from build123d import *

# Parameters (mm, degrees)
SKETCH_1_R               = 2
EXTRUDE_1_DEPTH          = 16
EXTRUDE_2_DEPTH          = 3
SKETCH_4_R               = 3.15
CUT_EXTRUDE_6_DEPTH      = 2.5
FILLET_3_R               = 0.6
SKETCH_7_R               = 3.175
EXTRUDE_3_DEPTH          = 1.4
CUT_EXTRUDE_9_DEPTH      = 1
CUT_EXTRUDE_9_DEPTH_BACK = 26
FILLET_6_R               = 1
EXTRUDE_5_DEPTH          = 3
FILLET_7_R               = 0.3
CUT_EXTRUDE_10_REACH     = 2.675
SKETCH_13_R              = 1.8
CUT_EXTRUDE_11_REACH     = 18
SKETCH_14_W              = 2.079062288
SKETCH_14_H              = 0.49177122


with BuildPart() as part:
    # Sketch 1 → Extrude 1 (new body)
    with BuildSketch(Plane(origin=(0, 0, 0), x_dir=(1, 0, 0), z_dir=(0, 1, 0))):
        Circle(SKETCH_1_R)
    extrude(amount=EXTRUDE_1_DEPTH)

    # Fillet 3
    fillet_3_edges = [part.edges().sort_by_distance(p)[0] for p in [
        (-2, 0, 0),
    ]]
    fillet(fillet_3_edges, radius=FILLET_3_R)

    # Sketch 7 → Extrude 3 (add)
    with BuildSketch(Plane(origin=(0, 16, 0), x_dir=(1, 0, 0), z_dir=(0, 1, 0))):
        Circle(SKETCH_7_R)
    extrude(amount=-EXTRUDE_3_DEPTH)

    # Sketch 10 → Cut-Extrude 9 (cut, two sides)
    with BuildSketch(Plane.XZ) as cut_extrude_9_sk:
        with BuildLine():
            Line((-1.307669683, 0.5), (1.307669683, 0.5))
            ThreePointArc((1.307669683, 0.5), (0, -1.4), (-1.307669683, 0.5))
        make_face()
    extrude(amount=CUT_EXTRUDE_9_DEPTH, mode=Mode.SUBTRACT)
    extrude(cut_extrude_9_sk.sketch, amount=-CUT_EXTRUDE_9_DEPTH_BACK, mode=Mode.SUBTRACT)

    # Fillet 6
    fillet_6_edges = [part.edges().sort_by_distance(p)[0] for p in [
        (0, 16, -1.4),
    ]]
    fillet(fillet_6_edges, radius=FILLET_6_R)



with BuildPart() as body_2:
    # Sketch 2 → Extrude 2 (new body)
    with BuildSketch(Plane.XY):
        with BuildLine():
            ThreePointArc((4.245738578, 21.991208882), (-3.671541908, 23.101880092), (0, 16))
            ThreePointArc((0, 16), (3.671541908, 17.898119908), (4.245738578, 21.991208882))
        make_face()
    extrude(amount=EXTRUDE_2_DEPTH)

    # Sketch 4 → Cut-Extrude 6 (cut)
    with BuildSketch(Plane(origin=(0, 0, 0), x_dir=(-1, 0, 0), z_dir=(0, 0, -1))):
        with Locations((0, 20.5)):
            Circle(SKETCH_4_R)
    extrude(amount=-CUT_EXTRUDE_6_DEPTH, mode=Mode.SUBTRACT)


with BuildPart() as part_1:
    add(part.part)

    add(body_2.part)  # Extrude 5 merges body 2
    # Sketch 12 → Extrude 5 (add)
    with BuildSketch(Plane.XY.offset(3)):
        with BuildLine():
            Line((-3.175, 16), (-4.239526881, 18.991221744))
            ThreePointArc((-4.239526881, 18.991221744), (0, 16), (4.239526881, 18.991221744))
            Line((4.239526881, 18.991221744), (3.175, 16))
            Line((3.175, 16), (3.175, 14.6))
            Line((3.175, 14.6), (-3.175, 14.6))
            Line((-3.175, 14.6), (-3.175, 16))
        make_face()
    extrude(amount=-EXTRUDE_5_DEPTH)

    # Fillet 7
    fillet_7_edges = [part_1.edges().sort_by_distance(p)[0] for p in [
        (3.15, 20.5, 0),
    ]]
    fillet(fillet_7_edges, radius=FILLET_7_R)

    # Sketch 13 → Cut-Extrude 10 (cut, up to next)
    with BuildSketch(Plane(origin=(0, 0, 2.5), x_dir=(-1, 0, 0), z_dir=(0, 0, -1)), mode=Mode.PRIVATE) as cut_extrude_10_sk1:
        with Locations((0, 20.5)):
            Circle(SKETCH_13_R)
    cut_extrude_10_tool1 = extrude(cut_extrude_10_sk1.sketch, amount=-CUT_EXTRUDE_10_REACH, mode=Mode.PRIVATE) & part_1.part
    add(cut_extrude_10_tool1.solids().sort_by_distance((0, 20.5, 2.5))[0], mode=Mode.SUBTRACT)

    # Sketch 14 → Cut-Extrude 11 (cut, up to next)
    with BuildSketch(Plane(origin=(0, 16, 0), x_dir=(1, 0, 0), z_dir=(0, 1, 0)), mode=Mode.PRIVATE) as cut_extrude_11_sk1:
        with Locations((0, -3.24588561)):
            Rectangle(SKETCH_14_W, SKETCH_14_H)
    cut_extrude_11_tool1 = extrude(cut_extrude_11_sk1.sketch, amount=-CUT_EXTRUDE_11_REACH, mode=Mode.PRIVATE) & part_1.part
    add(cut_extrude_11_tool1.solids().sort_by_distance((0, 16, 3.245886))[0], mode=Mode.SUBTRACT)


solid = part_1.part
Input: part model. Units: mm. Frame: model coordinates. A direction names the side the tool comes from. Give positions to 0.01 mm unless a question says otherwise; leave off trailing zeros. Order: outer loops, then holes, each group sorted by start corner. A loop starts at its lowest first (then second) coordinate and runs counter-clockwise, first axis right, second up. Notation, with made-up numbers: (-18, 12.5) -> (40, 12.5) arc R10 cw to (40, 21.5) -> close; hole circle Ø11 at (49.25, -0.75). An arc over 180 degrees is marked (long way). Use one line per item in the form item = value.
1) Section A-A, the plane x = 0. Return loops of the section in (y, z) (3 decimals).
Response values:
outline = (0, -1.4) arc R0.6 ccw to (0.6, -2) -> (14.6, -2) -> (14.6, -3.175) -> (16, -3.175) -> (16, -2.4) arc R1 ccw to (15, -1.4) -> close; (0, 0.5) -> (14.6, 0.5) -> (14.6, 0) -> (17.05, 0) arc R0.3 ccw to (17.35, 0.3) -> (17.35, 2.5) -> (18.7, 2.5) -> (18.7, 3) -> (14.6, 3) -> (14.6, 2) -> (0.6, 2) arc R0.6 ccw to (0, 1.4) -> close; (22.3, 2.5) -> (23.65, 2.5) -> (23.65, 0.3) arc R0.3 ccw to (23.95, 0) -> (25, 0) -> (25, 3) -> (22.3, 3) -> close
2) First-contact query: pin 1 Ø2 at (x, y) = (-0.5, 4) entering from -Z; pin 2 Ø5 at (x, y) = (1, 22.5) entering from -Z; pin 3 Ø1.1 at (y, z) = (15.5, 2) entering from +X; pin 4 Ø3 at (x, y) = (0, 20.5) entering from -Z. Flat tips, straight axial feed; report the tip coordinate or a pass-through.
Response values:
pin_1 = -2
pin_2 = 0
pin_3 = 3.19
pin_4 = through
3) Section B-B, the plane z = 2.75. Return loops of the section in (x, y) (3 decimals).
Response values:
outline = (-4.24, 18.991) -> (-3.175, 16) -> (-3.175, 14.6) -> (3.175, 14.6) -> (3.175, 16) -> (4.24, 18.991) arc R4.5 ccw (long way) to start; hole circle Ø3.6 at (0, 20.5)
4) Mould query, pull axis Y, two halves, no side actions, for faces 1 (the flat face through (3.715, 17.517, 1.521)), 2 (the flat face through (-1.4, 19.1, 2.5)), 3 (the cylindrical face through (0.234, 22.285, 2.746)), 4 (the cylindrical face through (0, 7.4, -1.4)). Classes: pulls with the +Y half, pulls with the -Y half, needs draft (parallel to the pull), parting line crosses it, or undercut.
Response values:
face_1 = pulls with the -Y half
face_2 = undercut
face_3 = undercut
face_4 = needs draft
5) Section D-D, the plane y = 6. Return loops of the section in (x, z).
Response values:
outline = circle Ø4 at (0, 0); hole (-1.31, 0.5) arc R1.4 ccw (long way) to (1.31, 0.5) -> close
6) Section C-C, the plane y = 20.5. Return loops of the section in (x, z).
Response values:
outline = (-4.5, 0) -> (-3.45, 0) arc R0.3 ccw to (-3.15, 0.3) -> (-3.15, 2.5) -> (-1.8, 2.5) -> (-1.8, 3) -> (-4.5, 3) -> close; (1.8, 2.5) -> (3.15, 2.5) -> (3.15, 0.3) arc R0.3 ccw to (3.45, 0) -> (4.5, 0) -> (4.5, 3) -> (1.8, 3) -> close
7) Reachability of faces 5 (the cylindrical face through (0.683, 17.425, 1.385)), 6 (the flat face through (0, 16, -3)), 7 (the cylindrical face through (0, 8, 2)), 8 (the flat face through (3.175, 15, 2)) from +Z, -Z, +X, -X, +Y, -Y: full face, straight path, thin tool, end or side. Return the list, or none.
Response values:
face_5 = -Z
face_6 = -Z, +X, -X, +Y
face_7 = -Y
face_8 = +Z, -Z, +X, -Y
8) Line query: probe 1 along Z at (x, y) = (0, 11.25); probe 2 along X at (y, z) = (4.75, 0); probe 3 along Y at (x, z) = (2.5, 1.5). Output: solid intervals per line, ascending.
Response values:
probe_1 = -2 to -1.4, 0.5 to 2
probe_2 = -2 to -1.4, 1.4 to 2
probe_3 = 14.6 to 18.58, 22.42 to 24.24
